Here's how the part is built. I have some questions about the finished solid (model axes, mm). Face numbers are marked on the shaded views. A direction names the side the tool comes from. Give positions to 0.01 mm unless a question says otherwise; leave off trailing zeros. Loops run counter-clockwise (first coordinate to the right, second up) from the corner with the lowest first, then second, coordinate; pieces in that order, holes last. Notation, with made-up numbers: (-35, -17.5) - (-26, -17.5) arc R19 ccw to (-26, -11.5) - close; hole circle Ø5 at (-11.75, 12). An arc over 180 degrees is marked (long way). Return JSON: item names as keys, results as strings. Group by question number.
(1) On a 3-axis mill with a long thin cutter (end or side, diameter ignored), from which of +Z, -Z, +X, -X, +Y, -Y can I reach the whole of each face in a straight line? I mean the marked faces 4 and 5. Say none if no direction works.
(2) I need wall thicknesses on probe 1 along Z at (x, y) = (0, -7.8); probe 2 along Z at (x, y) = (0, -9.25); probe 3 along Y at (x, z) = (0, 13). Which ranges of each line are inside material? Lowest first, please. Write a range as [from, to].
(3) If we section it at D-D (z = 29.5): State how many separate pieces and enclosed holes the cut face has, then the cut area to 3 significant figures.
(4) If we section it at A-A (z = 15.5): Please give me the cut outline in (x, y), then the cut area to 3 significant figures.
(5) If we section it at B-B (y = -17): Please give me the cut outline in (x, z).
(6) If we section it at C-C (x = -15.5): Please give me the cut outline in (y, z).
(7) For P1, Ø3, axis at x = -1, z = 29, coming from the +Y side; P2, Ø1, axis at y = 14.5, z = 25.5, coming from the +X side; P3, Ø2, axis at x = -14.5, y = 12, coming from the +Z side, each with a flat end and sliding along its axis, tell me the tip position at first contact or that it passes through.
(8) If we mould it in two halves opening along Y, with no side actions, what happens to the marked faces 1, 2 and 3? For each: released by +Y, released by -Y, zero draft, split by the parting line, or undercut.
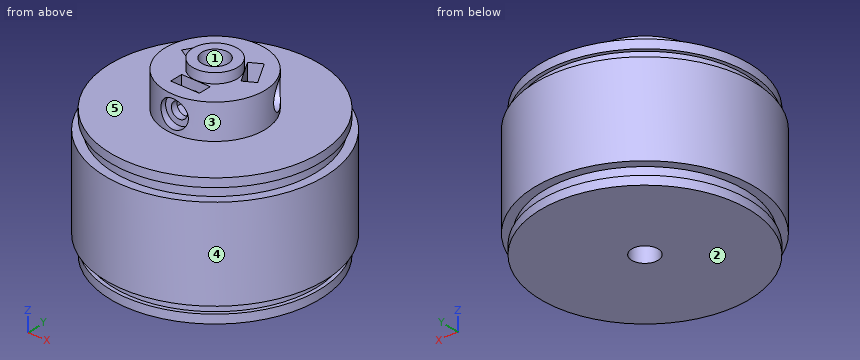
```python
from build123d import *

# Parameters (mm, degrees)
EXTRUDE_1_OUTLINE_R      = 22
EXTRUDE_1_DEPTH          = 26
SKETCH_2_W               = 1.75
SKETCH_2_H               = 1
SKETCH_2_W_2             = 2
SKETCH_2_H_2             = 1.75
SKETCH_3_R               = 2.65
CUT_EXTRUDE_1_DEPTH      = 41.546269865
EXTRUDE_START            = 7
SKETCH_4_R               = 10
SKETCH_4_R_2             = 2.65
EXTRUDE_2_DEPTH          = 7
SKETCH_5_R               = 1.6
CUT_EXTRUDE_2_DEPTH      = 46.354161882
CUT_EXTRUDE_START        = -8.5
SKETCH_6_R               = 2.75
SKETCH_6_R_2             = 1.6
CUT_EXTRUDE_3_DEPTH      = 9
CUT_EXTRUDE_START_2      = -9.45
CUT_EXTRUDE_4_OUTLINE_R  = 1.6
CUT_EXTRUDE_4_DEPTH      = 2.6
PATTERN_CIRCULAR_1_COUNT = 3
EXTRUDE_START_2          = 2
SKETCH_8_R               = 4.5
SKETCH_8_R_2             = 2.65
EXTRUDE_3_DEPTH          = 2


# Read off the part's stored shape, not the designer's step: Бобышка-Вытянуть1, Вырез-Вытянуть4
with BuildPart() as part:
    # Бобышка-Вытянуть1 outline → Бобышка-Вытянуть1 (new body)
    with BuildSketch(Plane.XY):
        Circle(EXTRUDE_1_OUTLINE_R)
    extrude(amount=EXTRUDE_1_DEPTH)

    # Эскиз2 → Вырез-Повернуть1 (revolve, cut)
    with BuildSketch(Plane(origin=(0, 0, 0), x_dir=(0, 0, -1), z_dir=(1, 0, 0)), mode=Mode.PRIVATE) as cut_revolve_1_sk:
        Polygon((-3.75, 22), (-3.75, 20.25), (-1.75, 20.25), (-1.75, 21), (-1.75, 22), align=None)
        Polygon((-24.25, 21), (-24.25, 20.25), (-22.25, 20.25), (-22.25, 22), (-24.25, 22), align=None)
        with Locations((-25.125, 21.5)):
            Rectangle(SKETCH_2_W, SKETCH_2_H)
        with Locations((-23.25, 21.125)):
            Rectangle(SKETCH_2_W_2, SKETCH_2_H_2)
        with Locations((-2.75, 21.125)):
            Rectangle(SKETCH_2_W_2, SKETCH_2_H_2)
        with Locations((-0.875, 21.5)):
            Rectangle(SKETCH_2_W, SKETCH_2_H)
    revolve(cut_revolve_1_sk.sketch.rotate(Axis((0, 0, 0), (0, 0, 1)), 90), axis=Axis((0, 0, 0), (0, 0, 1)), mode=Mode.SUBTRACT)

    # Эскиз3 → Вырез-Вытянуть1 (cut, through all)
    with BuildSketch(Plane.XY.offset(26)):
        Circle(SKETCH_3_R)
    extrude(amount=-CUT_EXTRUDE_1_DEPTH, mode=Mode.SUBTRACT)

    # Эскиз4 → Бобышка-Вытянуть2 (add)
    with BuildSketch(Plane.XY.offset(26).offset(EXTRUDE_START)):
        Circle(SKETCH_4_R)
        Circle(SKETCH_4_R_2, mode=Mode.SUBTRACT)
    extrude(amount=-EXTRUDE_2_DEPTH)

    # Эскиз5 → Вырез-Вытянуть2 (cut, through all)
    with BuildSketch(Plane(origin=(0, 0, 0), x_dir=(1, 0, 0), z_dir=(0, 1, 0))):
        with Locations(Location((0, -29.5, 0), (0, 0, 270))):
            Circle(SKETCH_5_R)
    cut_extrude_2 = extrude(amount=-CUT_EXTRUDE_2_DEPTH, mode=Mode.SUBTRACT)

    # Эскиз6 → Вырез-Вытянуть3 (cut)
    with BuildSketch(Plane(origin=(0, 0, 0), x_dir=(1, 0, 0), z_dir=(0, 1, 0)).offset(CUT_EXTRUDE_START)):
        with Locations(Location((0, -29.5, 0), (0, 0, 270))):
            Circle(SKETCH_6_R)
        with Locations(Location((0, -29.5, 0), (0, 0, 270))):
            Circle(SKETCH_6_R_2, mode=Mode.SUBTRACT)
    cut_extrude_3 = extrude(amount=-CUT_EXTRUDE_3_DEPTH, mode=Mode.SUBTRACT)

    # Вырез-Вытянуть4 outline → Вырез-Вытянуть4 (cut)
    with BuildSketch(Plane.XZ.offset(14).offset(CUT_EXTRUDE_START_2)):
        Polygon((-2.875, 27.840117976), (0, 26.180235952), (2.875, 27.840117976), (2.875, 33), (-2.875, 33), align=None)
        with Locations((0, 29.5)):
            Circle(CUT_EXTRUDE_4_OUTLINE_R, mode=Mode.SUBTRACT)
    cut_extrude_4 = extrude(amount=CUT_EXTRUDE_4_DEPTH, mode=Mode.SUBTRACT)

    # Круговой массив1: Вырез-Вытянуть2, Вырез-Вытянуть3, Вырез-Вытянуть4 ×3 about axis
    pattern_circular_1_axis = Axis((0, 0, 0), (0, 0, 1))
    add([cut_extrude_2.rotate(pattern_circular_1_axis, i * 360 / PATTERN_CIRCULAR_1_COUNT) for i in range(1, PATTERN_CIRCULAR_1_COUNT)], mode=Mode.SUBTRACT)
    add([cut_extrude_3.rotate(pattern_circular_1_axis, i * 360 / PATTERN_CIRCULAR_1_COUNT) for i in range(1, PATTERN_CIRCULAR_1_COUNT)], mode=Mode.SUBTRACT)
    add([cut_extrude_4.rotate(pattern_circular_1_axis, i * 360 / PATTERN_CIRCULAR_1_COUNT) for i in range(1, PATTERN_CIRCULAR_1_COUNT)], mode=Mode.SUBTRACT)

    # Эскиз8 → Бобышка-Вытянуть3 (add)
    with BuildSketch(Plane.XY.offset(33).offset(EXTRUDE_START_2)):
        Circle(SKETCH_8_R)
        Circle(SKETCH_8_R_2, mode=Mode.SUBTRACT)
    extrude(amount=-EXTRUDE_3_DEPTH)


solid = part.part
```
Values:
{
 "1": {"face 4": "+Z, -Z", "face 5": "+Z"},
 "2": {"probe 1": "[0, 27.9], [31.1, 33]", "probe 2": "[0, 26.75], [32.25, 33]", "probe 3": "[-22, -2.65], [2.65, 22]"},
 "3": {"separate pieces": "3", "enclosed holes": "0", "area": "192 mm2"},
 "4": {"outline": "circle Ø44 at (0, 0); hole circle Ø5.3 at (0, 0)", "area": "1,500 mm2"},
 "5": {"outline": "(-13.96, 3.75) - (-11, 3.75) - (-11, 1.75) - (-12.33, 1.75) - (-12.33, 0) - (12.33, 0) - (12.33, 1.75) - (11, 1.75) - (11, 3.75) - (13.96, 3.75) - (13.96, 22.25) - (11, 22.25) - (11, 24.25) - (12.33, 24.25) - (12.33, 26) - (-12.33, 26) - (-12.33, 24.25) - (-11, 24.25) - (-11, 22.25) - (-13.96, 22.25) - close"},
 "6": {"outline": "(-15.61, 3.75) - (-13.03, 3.75) - (-13.03, 1.75) - (-14.17, 1.75) - (-14.17, 0) - (14.17, 0) - (14.17, 1.75) - (13.03, 1.75) - (13.03, 3.75) - (15.61, 3.75) - (15.61, 22.25) - (13.03, 22.25) - (13.03, 24.25) - (14.17, 24.25) - (14.17, 26) - (-14.17, 26) - (-14.17, 24.25) - (-13.03, 24.25) - (-13.03, 22.25) - (-15.61, 22.25) - close"},
 "7": {"P1": "y = 10", "P2": "x = 15.65", "P3": "z = 26"},
 "8": {"face 1": "undercut", "face 2": "zero draft", "face 3": "split by the parting line"}
}
